Source: CAD feature listing. Evaluate the final solid. Frame: model axes, mm. A direction names the side the tool comes from. Round coordinates to 2 decimals unless told otherwise and drop trailing zeros. Write each loop counter-clockwise with the first axis right and the second up, starting at its lowest first coordinate (ties: lowest second). Pieces come first, ordered by that corner, then holes. Notation, with made-up numbers: M -25.5,-4 L 17.5,-4 A8 cw 17.5,3 Z; hole C 86,10 d9. An arc over 180 degrees is marked long. Put each result on its own line as item: value. Start each with the question number.
```python
from build123d import *

# Parameters (mm, degrees)
F0_R     = 3
F0_R_2   = 7.5
F1_DEPTH = 10


with BuildPart() as f1:
    # F0 (on Front) → F1 (new body)
    with BuildSketch(Plane.XZ):
        with BuildLine():
            Line((-13.302721, 26.889359), (-12.269592, 21.782037))
            ThreePointArc((-12.269592, 21.782037), (-13.889256, 20.78674), (-15.428608, 19.671249))
            Line((-15.428608, 19.671249), (-19.751797, 22.580224))
            ThreePointArc((-19.751797, 22.580224), (-21.213203, 21.213203), (-22.580224, 19.751797))
            Line((-22.580224, 19.751797), (-19.671249, 15.428608))
            ThreePointArc((-19.671249, 15.428608), (-20.78674, 13.889256), (-21.782037, 12.269592))
            Line((-21.782037, 12.269592), (-26.889359, 13.302721))
            ThreePointArc((-26.889359, 13.302721), (-27.716386, 11.480503), (-28.420092, 9.607203))
            Line((-28.420092, 9.607203), (-24.078137, 6.726314))
            ThreePointArc((-24.078137, 6.726314), (-24.519632, 4.877258), (-24.819347, 3))
            Line((-24.819347, 3), (-29.933259, 2))
            ThreePointArc((-29.933259, 2), (-30, 0), (-29.933259, -2))
            Line((-29.933259, -2), (-24.819347, -3))
            ThreePointArc((-24.819347, -3), (-24.519632, -4.877258), (-24.078137, -6.726314))
            Line((-24.078137, -6.726314), (-28.420092, -9.607203))
            ThreePointArc((-28.420092, -9.607203), (-27.716386, -11.480503), (-26.889359, -13.302721))
            Line((-26.889359, -13.302721), (-21.782037, -12.269592))
            ThreePointArc((-21.782037, -12.269592), (-20.78674, -13.889256), (-19.671249, -15.428608))
            Line((-19.671249, -15.428608), (-22.580224, -19.751797))
            ThreePointArc((-22.580224, -19.751797), (-21.213203, -21.213203), (-19.751797, -22.580224))
            Line((-19.751797, -22.580224), (-15.428608, -19.671249))
            ThreePointArc((-15.428608, -19.671249), (-13.889256, -20.78674), (-12.269592, -21.782037))
            Line((-12.269592, -21.782037), (-13.302721, -26.889359))
            ThreePointArc((-13.302721, -26.889359), (-11.480503, -27.716386), (-9.607203, -28.420092))
            Line((-9.607203, -28.420092), (-6.726314, -24.078137))
            ThreePointArc((-6.726314, -24.078137), (-4.877258, -24.519632), (-3, -24.819347))
            Line((-3, -24.819347), (-2, -29.933259))
            ThreePointArc((-2, -29.933259), (0, -30), (2, -29.933259))
            Line((2, -29.933259), (3, -24.819347))
            ThreePointArc((3, -24.819347), (4.877258, -24.519632), (6.726314, -24.078137))
            Line((6.726314, -24.078137), (9.607203, -28.420092))
            ThreePointArc((9.607203, -28.420092), (11.480503, -27.716386), (13.302721, -26.889359))
            Line((13.302721, -26.889359), (12.269592, -21.782037))
            ThreePointArc((12.269592, -21.782037), (13.889256, -20.78674), (15.428608, -19.671249))
            Line((15.428608, -19.671249), (19.751797, -22.580224))
            ThreePointArc((19.751797, -22.580224), (21.213203, -21.213203), (22.580224, -19.751797))
            Line((22.580224, -19.751797), (19.671249, -15.428608))
            ThreePointArc((19.671249, -15.428608), (20.78674, -13.889256), (21.782037, -12.269592))
            Line((21.782037, -12.269592), (26.889359, -13.302721))
            ThreePointArc((26.889359, -13.302721), (27.716386, -11.480503), (28.420092, -9.607203))
            Line((28.420092, -9.607203), (24.078137, -6.726314))
            ThreePointArc((24.078137, -6.726314), (24.519632, -4.877258), (24.819347, -3))
            Line((24.819347, -3), (29.933259, -2))
            ThreePointArc((29.933259, -2), (30, 0), (29.933259, 2))
            Line((29.933259, 2), (24.819347, 3))
            ThreePointArc((24.819347, 3), (24.519632, 4.877258), (24.078137, 6.726314))
            Line((24.078137, 6.726314), (28.420092, 9.607203))
            ThreePointArc((28.420092, 9.607203), (27.716386, 11.480503), (26.889359, 13.302721))
            Line((26.889359, 13.302721), (21.782037, 12.269592))
            ThreePointArc((21.782037, 12.269592), (20.78674, 13.889256), (19.671249, 15.428608))
            Line((19.671249, 15.428608), (22.580224, 19.751797))
            ThreePointArc((22.580224, 19.751797), (21.213203, 21.213203), (19.751797, 22.580224))
            Line((19.751797, 22.580224), (15.428608, 19.671249))
            ThreePointArc((15.428608, 19.671249), (13.889256, 20.78674), (12.269592, 21.782037))
            Line((12.269592, 21.782037), (13.302721, 26.889359))
            ThreePointArc((13.302721, 26.889359), (11.480503, 27.716386), (9.607203, 28.420092))
            Line((9.607203, 28.420092), (6.726314, 24.078137))
            ThreePointArc((6.726314, 24.078137), (4.877258, 24.519632), (3, 24.819347))
            Line((3, 24.819347), (2, 29.933259))
            ThreePointArc((2, 29.933259), (0, 30), (-2, 29.933259))
            Line((-2, 29.933259), (-3, 24.819347))
            ThreePointArc((-3, 24.819347), (-4.877258, 24.519632), (-6.726314, 24.078137))
            Line((-6.726314, 24.078137), (-9.607203, 28.420092))
            ThreePointArc((-9.607203, 28.420092), (-11.480503, 27.716386), (-13.302721, 26.889359))
        make_face()
        with Locations((-8.816779, -12.135255)):
            Circle(F0_R, mode=Mode.SUBTRACT)
        with Locations((8.816779, -12.135255)):
            Circle(F0_R, mode=Mode.SUBTRACT)
        with Locations((-14.265848, 4.635255)):
            Circle(F0_R, mode=Mode.SUBTRACT)
        Circle(F0_R_2, mode=Mode.SUBTRACT)
        with Locations((14.265848, 4.635255)):
            Circle(F0_R, mode=Mode.SUBTRACT)
        with Locations((0, 15)):
            Circle(F0_R, mode=Mode.SUBTRACT)
    extrude(amount=F1_DEPTH)


solid = f1.part
```
(1) Access query for faces 1 (the flat face through (-27.412, -4.93, -2.493)), 2 (the flat face through (27.341, -4.93, -2.507)), 3 (the flat face through (-17.62, -4.93, -21.146)), 4 (the cylindrical face through (21.193, -4.93, -21.233)), 5 (the cylindrical face through (13.911, -4.93, 20.772)). Directions: +Z, -Z, +X, -X, +Y, -Y. A direction counts if a zero-diameter tool reaches every point of the face in a straight line with its end or side. Return the directions, or none.
(2) Contact query for flat-ended pins moving along their axis: P1, Ø2, axis at y = -4.5, z = 14, coming from the +X side; P2, Ø3, axis at y = -4.5, z = -20, coming from the -X side; P3, Ø5, axis at x = 8.5, y = -8.5, coming from the +Z side. Output: stop coordinate, or through.
(3) Section query B-B (z = 0). Return loops of the section in (x, y).
(4) Ray query, line 1 along Z through (x, y) = (0, -3); line 2 along Z through (x, y) = (-1.5, -8.75); line 3 along X through (y, z) = (-7, 4). Return the intervals inside material, ascending.
(5) Section query C-C (y = -6.25). Count the separate pieces of the cut face and the enclosed holes in it, and give its area (3 significant figures).
(6) Section query A-A (x = 0). Return loops of the section in (y, z).
(7) Pull-direction query (Z, two-part tool) for faces 6 (the flat face through (17.62, -4.93, 21.146)), 7 (the cylindrical face through (4.851, -4.93, -24.525)), 8 (the cylindrical face through (-24.525, -4.93, -4.851)); classes: +Z half, -Z half, draft (parallel to the pull), parting line (faces both ways), or undercut.
Entries:
1. face 1: -X, +Y, -Y
1. face 2: +X, +Y, -Y
1. face 3: -Z, +Y, -Y
1. face 4: -Z, +X, +Y, -Y
1. face 5: +Y, -Y
2. P1: x = 27.04
2. P2: x = -22.58
2. P3: z = 28.42
3. outline: M -30,-10 L -7.5,-10 L -7.5,0 L -30,0 Z; M 7.5,-10 L 30,-10 L 30,0 L 7.5,0 Z
4. line 1: -30 to -7.5, 7.5 to 12, 18 to 30
4. line 2: -29.96 to -7.35, 7.35 to 12.4, 17.6 to 29.96
4. line 3: -24.68 to -17.2, -11.33 to -6.34, 6.34 to 11.33, 17.2 to 24.68
5. separate pieces: 1
5. enclosed holes: 6
5. area: 2,050 mm2
6. outline: M -10,-30 L 0,-30 L 0,-7.5 L -10,-7.5 Z; M -10,7.5 L 0,7.5 L 0,12 L -10,12 Z; M -10,18 L 0,18 L 0,30 L -10,30 Z
7. face 6: +Z half
7. face 7: -Z half
7. face 8: undercut
